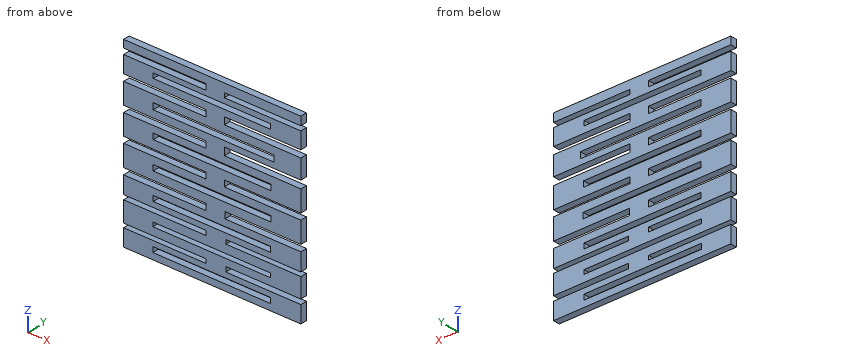
from build123d import *

# Parameters (mm, degrees)
F0_W     = 89.507591
F0_H     = 4.047405
F0_H_2   = 3.206663
F0_W_2   = 89.219786
F0_H_3   = 4.051941
F0_W_3   = 89.795395
F0_H_4   = 4.339748
F0_H_5   = 4.34881
F0_W_4   = 89.131403
F0_H_6   = 3.709744
F0_W_5   = 91.964136
F0_H_7   = 4.813378
F1_DEPTH = 5


with BuildPart() as f1:
    # F0 (on Front) → F1 (new body)
    with BuildSketch(Plane.XZ):
        Polygon((64.727969, 69.582537), (-70.183687, 69.582537), (-70.183687, 63.748978), (-7.506745, 63.748978), (-7.506745, 59.431892), (-70.183687, 59.431892), (-70.183687, 46.48063), (-7.506745, 46.48063), (-7.506745, 41.499555), (-70.183687, 41.499555), (-70.183687, 25.47081), (-7.506745, 25.47081), (-7.506745, 20.564513), (-70.183687, 20.564513), (-70.183687, 4.67401), (-7.506745, 4.67401), (-7.603418, 0), (-70.183687, 0), (-70.183687, -16.288219), (-7.506745, -16.288219), (-7.506745, -21.103866), (-70.183687, -21.103866), (-70.183687, -34.392789), (-7.626853, -34.392789), (-7.506745, -37.816998), (-70.183687, -37.816998), (-70.183687, -53.38797), (-7.626853, -53.38797), (-7.506745, -56.513045), (-70.183687, -56.513045), (-70.183687, -69.527753), (64.727969, -69.527753), (64.727969, -56.513045), (7.626853, -56.513045), (7.626853, -52.81236), (64.727969, -52.81236), (64.727969, -37.816998), (7.626853, -37.816998), (7.626853, -34.680594), (64.727969, -34.680594), (64.727969, -21.185448), (7.051241, -21.185448), (7.051241, -16.288219), (64.727969, -16.288219), (64.727969, 0), (6.47563, 0), (6.47563, 4.67401), (64.727969, 4.67401), (64.727969, 20.905621), (6.47563, 20.905621), (6.47563, 26.769336), (64.727969, 26.769336), (64.727969, 41.574333), (6.47563, 41.574333), (6.47563, 47.056243), (64.727969, 47.056243), (64.727969, 59.719693), (6.47563, 59.719693), (6.47563, 63.173369), (64.727969, 63.173369), align=None)
        with Locations((-3.165862, -62.606814)):
            Rectangle(F0_W, F0_H, mode=Mode.SUBTRACT)
        with Locations((-3.165862, -45.781515)):
            Rectangle(F0_W, F0_H_2, mode=Mode.SUBTRACT)
        with Locations((-3.021959, -28.360198)):
            Rectangle(F0_W_2, F0_H_3, mode=Mode.SUBTRACT)
        with Locations((-2.734154, -7.782086)):
            Rectangle(F0_W_3, F0_H_4, mode=Mode.SUBTRACT)
        with Locations((-2.878056, 13.223202)):
            Rectangle(F0_W, F0_H_5, mode=Mode.SUBTRACT)
        with Locations((-3.06615, 53.835543)):
            Rectangle(F0_W_4, F0_H_6, mode=Mode.SUBTRACT)
        with Locations((-1.649784, 33.425127)):
            Rectangle(F0_W_5, F0_H_7, mode=Mode.SUBTRACT)
    extrude(amount=F1_DEPTH)


solid = f1.part
Design review of the part built by this model. Coordinates are the model's own, in mm. Give positions to 0.01 mm unless a question says otherwise; leave off trailing zeros. Write each loop counter-clockwise with the first axis right and the second up, starting at its lowest first coordinate (ties: lowest second). Pieces come first, ordered by that corner, then holes. Notation, with made-up numbers: M 51,-19 L 106,-19 A23 cw 106,-8 Z; hole C 12.25,75 d1. An arc over 180 degrees is marked long. Return JSON: item names as keys, results as strings. Group by question number.
Item 1: Wall thickness on line 1 along X through (y, z) = (-2.35, 11.5); line 2 along X through (y, z) = (-2.6, -47); line 3 along X through (y, z) = (-4.4, 26): over which ranges is each line inside the solid? List them lowest first.
Item 2: Take a section at A-A (x = 53). Count the separate pieces of the cut face and the enclosed holes in it, plus the area to 3 significant figures.
Item 3: Take a section at D-D (z = -18). Give the boundary of the cut face in (x, y).
Item 4: Clearance check with flat-ended pins moving along their axes: pin 1 Ø1.9 at (y, z) = (-2.5, -55) entering from +X; pin 2 Ø1 at (y, z) = (-1, 3) entering from -X. State where each tip first meets the part, or that it passes through.
Return value:
{
 "1": {"line 1": "x = -70.18 to -47.63, 41.88 to 64.73", "line 2": "x = -70.18 to -47.92, 41.59 to 64.73", "line 3": "x = -70.18 to 6.48"},
 "2": {"separate pieces": "8", "enclosed holes": "0", "area": "540 mm2"},
 "3": {"outline": "M -7.51,-5 L 7.05,-5 L 7.05,0 L -7.51,0 Z"},
 "4": {"pin 1": "stops at x = 7.63", "pin 2": "stops at x = -7.55"}
}
